Input: part model. Units: mm. Frame: model coordinates. Face numbers are marked on the shaded views. A direction names the side the tool comes from. Round coordinates to 2 decimals unless told otherwise and drop trailing zeros. Order: outer loops, then holes, each group sorted by start corner. A loop starts at its lowest first (then second) coordinate and runs counter-clockwise, first axis right, second up.
Item 1: Line query: L1, parallel to Z at x = 0, y = 4; L2, parallel to X at y = 12.5, z = 4.5; L3, parallel to X at y = 17, z = -1.25. Output: solid intervals per line, ascending.
Item 2: Reachability of the marked faces 1 and 2 from +Z, -Z, +X, -X, +Y, -Y: full face, straight path, thin tool, end or side. Return the list, or none.
Item 3: Cut plane A-A on y = 3. Output: boundary loops of the cut face in (x, z).
Item 4: First-contact query: pin 1 (5.5 mm diameter, centred on x = 0, z = 0, fed in from +Y); pin 2 (5 mm diameter, centred on y = 8, z = 3.5, fed in from +X); pin 3 (4 mm diameter, centred on x = 39.5, z = 3, fed in from -Y). Flat tips, straight axial feed; report the tip coordinate or a pass-through.
Item 5: Cut plane B-B on x = 41.5. Output: boundary loops of the cut face in (y, z), then the cut area to 3 significant figures.
Autodesk Inventor part; units mm, degrees
ref_plane "RR_XY" through (60, 32, 0) normal (1, 0, 0) x (0, 0, -1)
ref_plane "RR_YZ" through (60, 32, 0) normal (0, 0, -1) x (0, 1, 0)
ref_plane "RR_ZX" through (60, 32, 0) normal (0, 1, 0) x (1, 0, 0)
sketch "Sketch_1" plane through (0, 0, 0) normal (0, 0, 1) x (1, 0, 0)
  line L0 (0, 0) -> (0, 22)
  line L1 (0, 22) -> (5, 22)
  line L2 (5, 22) -> (5, 0)
  line L3 (5, 0) -> (0, 0)
  line L4 (0, 0) -> (0, 22)
revolve "Revolution1" add sketch "Sketch_1" angle 360 about axis through (0, 0, 0) along (0, -1, 0)
sketch "Sketch_2" plane through (0, 22, 0) normal (0, 1, 0) x (1, 0, 0)
  line L0 (10, 10) -> (10, -10)
  circle A0 centre (0, 0) radius 5
revolve "Revolution2" add sketch "Sketch_2" angle 90 about axis through (10, 22, -10) along (0, 0, -1)
sketch "Sketch3" plane through (0, 0, 0) normal (0, -1, 0) x (1, 0, 0)
  point P0 (0, 0)
hole "Hole1" at (0, 0, 0) direction (0, 1, 0) diameter 4.134 depth 12.4 tip angle 120 countersink diameter 5 countersink angle 90
sketch "Sketch_4" plane through (0, 0, 0) normal (0, 0, 1) x (1, 0, 0)
  line L0 (110, 32) -> (10, 32)
  line L1 (10, 32) -> (10, 37)
  line L2 (10, 37) -> (110, 37)
  line L3 (110, 37) -> (110, 32)
  line L4 (110, 32) -> (10, 32)
revolve "Revolution3" add sketch "Sketch_4" angle 360 about axis through (110, 32, 0) along (1, 0, 0)
sketch "Sketch_6" plane through (0, 22, 0) normal (0, 1, 0) x (1, 0, 0)
  line L0 (110, -10) -> (110, 10)
  circle A0 centre (120, 0) radius 5
revolve "Revolution4" add sketch "Sketch_6" angle 90 about axis through (110, 22, 10) along (0, 0, 1)
sketch "Sketch_5" plane through (0, 0, 0) normal (0, 0, 1) x (1, 0, 0)
  line L0 (120, 0) -> (120, 22)
  line L1 (120, 22) -> (125, 22)
  line L2 (125, 22) -> (125, 0)
  line L3 (125, 0) -> (120, 0)
  line L4 (120, 0) -> (120, 22)
revolve "Revolution5" add sketch "Sketch_5" angle 360 about axis through (120, 0, 0) along (0, -1, 0)
sketch "Sketch7" plane through (120, 0, 0) normal (0, -1, 0) x (1, 0, 0)
  point P0 (0, 0)
hole "Hole2" at (120, 0, 0) direction (0, 1, 0) diameter 4.134 depth 12 tip angle 120 countersink diameter 5 countersink angle 90
ref_plane "RR_XY" through (60, 32, 0) normal (1, 0, 0) x (0, 0, -1)
ref_plane "RR_YZ" through (60, 32, 0) normal (0, 0, -1) x (0, 1, 0)
ref_plane "RR_ZX" through (60, 32, 0) normal (0, 1, 0) x (1, 0, 0)
ref_plane "U_XY" through (0, 0, 0) normal (0, 1, 0) x (1, 0, 0)
ref_plane "U_YZ" through (0, 0, 0) normal (1, 0, 0) x (0, 0, -1)
ref_plane "U_ZX" through (0, 0, 0) normal (0, 0, -1) x (0, 1, 0)
ref_plane "U1_XY" through (120, 0, 0) normal (0, 1, 0) x (1, 0, 0)
ref_plane "U1_YZ" through (120, 0, 0) normal (1, 0, 0) x (0, 0, -1)
ref_plane "U1_ZX" through (120, 0, 0) normal (0, 0, -1) x (0, 1, 0)
properties part number "UWANK10-120-27" material "鋼、炭素鋼"
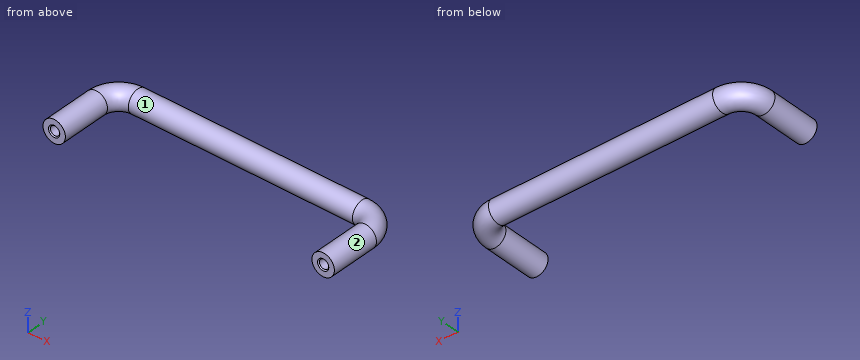
From the geometry:
1. L1: z = -5 to -2.07, 2.07 to 5
1. L2: x = -2.18 to 2.18, 117.82 to 122.18
1. L3: x = -4.84 to 4.84, 115.16 to 124.84
2. face 1: none
2. face 2: -Y
3. outline: circle Ø10 at (0, 0); circle Ø10 at (120, 0); hole circle Ø4.13 at (0, 0); hole circle Ø4.13 at (120, 0)
4. pin 1: stops at y = 35.13
4. pin 2: stops at x = 124.9
4. pin 3: stops at y = 27.1
5. outline: circle Ø10 at (32, 0)
5. area: 78.5 mm2
